For this review, take the finished solid that the model builds, in its own axes (mm). Coordinates: 2 decimals unless noted, no trailing zeros. Write each loop counter-clockwise with the first axis right and the second up, starting at its lowest first coordinate (ties: lowest second). Pieces come first, ordered by that corner, then holes. Notation, with made-up numbers: (54, 82.5) - (88, 82.5) arc R20 cw to (88, 121.5) - close; hole circle Ø1 at (53.5, 54.5). An arc over 180 degrees is marked (long way). Use one line per item in the form item = value. Start each with the question number.
1) We need section B-B (x = 13). Give the boundary of the cut face in (y, z), plus the area to 3 significant figures.
2) We need section A-A (z = -6.5). Give the boundary of the cut face in (x, y).
3) We need section C-C (x = 34.5). Give the boundary of the cut face in (y, z).
4) For L1, parallel to Y at x = 0, z = -4; L2, parallel to Y at x = 18.5, z = 3; L3, parallel to X at y = -43.5, z = -3.5, list the stretches that pass through material, from the lowest coordinate up. Write a range as from..to.
5) We need section D-D (y = 86). Give the boundary of the cut face in (x, z).
6) Mouldability with a two-part tool opening along Y and no side actions: class faces 1 (the cylindrical face through (23.846, 7.509, -0.14)), 2 (the flat face through (-20.213, 89.99, 0.14)), 3 (the flat face through (-1, 31, 10)), 4 (the cylindrical face through (-29.32, 12.23, 0.14)) as pulls with the +Y half, pulls with the -Y half, needs draft (parallel to the pull), parting line crosses it, or undercut.
7) Insertion check: P1, Ø1, axis at x = -42, z = 0, coming from the -Y side; P2, Ø8, axis at x = -57, z = 5, coming from the -Y side; P3, Ø6, axis at x = 49, z = 6.5, coming from the -Y side. Each pin has a flat end and moves straight along its axis. Give the tip position at first contact, or say it passes through.
```python
from build123d import *

# Parameters (mm, degrees)
SKETCH1_R           = 25
BOSS_EXTRUDE1_DEPTH = 10


with BuildPart() as part:
    # Sketch1 → Boss-Extrude1 (new body, symmetric)
    with BuildSketch(Plane.XY):
        with BuildLine():
            Line((41, 53.98591689), (0, 125))
            Line((0, 125), (-41, 53.98591689))
            ThreePointArc((-41, 53.98591689), (-29.653041557, 11.639425428), (-71.999407886, 0.292000007))
            ThreePointArc((-71.999407886, 0.292000007), (-60.81182851, -38.5476525), (-30.460070741, -65.23943662))
            ThreePointArc((-30.460070741, -65.23943662), (0, -40), (30.460070741, -65.23943662))
            ThreePointArc((30.460070741, -65.23943662), (60.81182851, -38.5476525), (71.999407886, 0.292000007))
            ThreePointArc((71.999407886, 0.292000007), (29.653041557, 11.639425428), (41, 53.98591689))
        make_face()
        Circle(SKETCH1_R, mode=Mode.SUBTRACT)
    extrude(amount=BOSS_EXTRUDE1_DEPTH, both=True)


solid = part.part
```
Determined:
q1.outline = (-42.86, -10) - (-21.35, -10) - (-21.35, 10) - (-42.86, 10) - close; (21.35, -10) - (102.48, -10) - (102.48, 10) - (21.35, 10) - close
q1.area = 2,050 mm²
q2.outline = (-72, 0.29) arc R72 ccw to (-30.46, -65.24) arc R31 cw to (30.46, -65.24) arc R72 ccw to (72, 0.29) arc R31 cw to (41, 53.99) - (0, 125) - (-41, 53.99) arc R31 cw to start; hole circle Ø50 at (0, 0)
q3.outline = (-63.2, -10) - (5.3, -10) - (5.3, 10) - (-63.2, 10) - close; (48.98, -10) - (65.24, -10) - (65.24, 10) - (48.98, 10) - close
q4.L1 = -40..-25, 25..125
q4.L2 = -46.13..-16.82, 16.82..92.96
q4.L3 = -57.37..-14.31, 14.31..57.37
q5.outline = (-22.52, -10) - (22.52, -10) - (22.52, 10) - (-22.52, 10) - close
q6.face_1 = undercut
q6.face_2 = pulls with the +Y half
q6.face_3 = needs draft
q6.face_4 = undercut
q7.P1 = -58.84
q7.P2 = -48.73
q7.P3 = -55.39
